The model under review builds one solid part; all positions refer to its coordinate system, in mm. Round coordinates to 2 decimals unless told otherwise and drop trailing zeros. Loops run counter-clockwise (first coordinate to the right, second up) from the corner with the lowest first, then second, coordinate; pieces in that order, holes last. Notation, with made-up numbers: (-14, -24) -> (22, -24) arc R25 ccw to (22, 5) -> close; hole circle Ø10 at (65.5, 55). An arc over 180 degrees is marked (long way). Use CSV: the item, a comma, the result in double quotes. Start each with the question number.
Autodesk Inventor part; units mm, degrees
ref_plane "YZ Plane" through (0, 0, 0) normal (1, 0, 0) x (0, 1, 0)
ref_plane "XZ Plane" through (0, 0, 0) normal (0, 1, 0) x (-1, 0, 0)
ref_plane "XY Plane" through (0, 0, 0) normal (0, 0, 1) x (1, 0, 0)
sketch "Skizze1" plane through (0, 0, 0) normal (1, 0, 0) x (0, 1, 0)
  line L0 (-50, -37.5) -> (50, -37.5)
  line L1 (50, -37.5) -> (50, 37.5)
  line L2 (50, 37.5) -> (-50, 37.5)
  line L3 (-50, 37.5) -> (-50, -37.5)
  line L4 (-50, -37.5) -> (50, 37.5) construction
  line L5 (50, -37.5) -> (-50, 37.5) construction
  point P0 (0, 0)
  dimension "d0" = 100
  dimension "d1" = 75
extrude "Extrusion1" add sketch "Skizze1" along normal blind 0.8
sketch "Skizze2" plane through (0.8, 0, 0) normal (1, 0, 0) x (0, 0, -1)
  line L0 (-37.5, -50) -> (-6.5, -50)
  line L1 (-6.5, -50) -> (-6.5, -44)
  line L2 (-6.5, -44) -> (-37.5, -44)
  line L3 (-37.5, -44) -> (-37.5, -50)
  line L4 (-37.5, 50) -> (-6.5, 50)
  line L5 (-6.5, 50) -> (-6.5, 44)
  line L6 (-6.5, 44) -> (-37.5, 44)
  line L7 (-37.5, 44) -> (-37.5, 50)
  line L8 (31.5, -50) -> (37.5, -50)
  line L9 (37.5, -50) -> (37.5, -44)
  line L10 (37.5, -44) -> (31.5, -44)
  line L11 (31.5, -44) -> (31.5, -50)
  line L12 (37.5, 50) -> (31.5, 50)
  line L13 (31.5, 50) -> (31.5, 44)
  line L14 (31.5, 44) -> (37.5, 44)
  line L15 (37.5, 44) -> (37.5, 50)
  line L16 (-2.5, -37.5) -> (27.5, -37.5)
  line L17 (27.5, -37.5) -> (27.5, 37.5)
  line L18 (27.5, 37.5) -> (-2.5, 37.5)
  line L19 (-2.5, 37.5) -> (-2.5, -37.5)
  line L20 (52.5, 0) -> (-52.5, 0) construction
  line L21 (-37.5, 50) -> (-37.5, -50) construction
  point P0 (0, 0)
  dimension "d4" = 6
  dimension "d5" = 6
  dimension "d6" = 31
  dimension "d9" = 75
  dimension "d10" = 30
  dimension "d11" = 35
extrude "Extrusion2" cut sketch "Skizze2" against normal through all
fillet "Rundung1" radius 6 6 edges at (0.4, -44, 6.5) (0.4, -44, -31.5) (0.4, 44, -31.5) (0.4, 44, 6.5) (0.4, 44, 37.5) (0.4, -44, 37.5)
fillet "Rundung1" radius 0.5 4 edges at (0.4, -37.5, 2.5) (0.4, -37.5, -27.5) (0.4, 37.5, -27.5) (0.4, 37.5, 2.5)
sketch "Skizze3" plane through (0.8, 0, 0) normal (1, 0, 0) x (0, 0, -1)
  line L0 (-37.5, 50) -> (95.7584, 50) construction
  line L1 (95.7584, 50) -> (95.7584, -50) construction
  line L2 (95.7584, -50) -> (-37.5, -50) construction
  line L3 (-37.5, -50) -> (-37.5, 50) construction
  line L4 (-6.5, -50) -> (31.5, -50)
  line L5 (-37.5, 38) -> (-37.5, -38)
  point P0 (0, 0)
  dimension "d26" = 100
decal "Aufkleber1"
sketch "Skizze4" plane through (0.8, 0, 0) normal (1, 0, 0) x (0, 0, -1)
  circle A0 centre (-31, -37.5) radius 1.25
  circle A1 centre (-31, 37.5) radius 1.25
  circle A2 centre (29, -41.5) radius 1.25
  circle A3 centre (29, 41.5) radius 1.25
  line L0 (-37.5, 38) -> (-37.5, -38)
  line L1 (-31.5, -44) -> (-12.5, -44)
  line L2 (52.5, 0) -> (-52.5, 0) construction
  line L3 (-6.5, -50) -> (31.5, -50) construction
  line L4 (37.5, -44) -> (37.5, 44) construction
  point P0 (0, 0)
  dimension "d32" = 6.5
  dimension "d33" = 6.5
  dimension "d34" = 2.5
  dimension "d35" = 8.5
  dimension "d36" = 8.5
extrude "Extrusion3" cut sketch "Skizze4" against normal through all
properties part number "EW_MessingplatteUhrzeit" material "Messing"
1. For line 1 along Y through (x, z) = (0.2, -29); line 2 along Y through (x, z) = (0.5, 31); line 3 along Y through (x, z) = (0.2, -25.5), list the stretches that pass through material, from the lowest coordinate up. Write a range as from..to.
2. Take a section at B-B, the plane z = -14. Give the boundary of the cut face in (x, y).
3. The part is to be moulded in two halves that separate along Z. For faces 1 (the face through (0, -1, 9)), 2 (the face through (0.394, -42.289, 35.696)), 3 (the face through (0.406, 37.021, 29.845)), 4 (the face through (0.41, 42.74, -28.84)), say which applies: pulls with the +Z half, pulls with the -Z half, needs draft (parallel to the pull), parting line crosses it, or undercut.
4. Take a section at C-C, the plane y = -9.5. Give the boundary of the cut face in (x, z), then the cut area to 3 significant figures.
5. Take a section at D-D, the plane x = 0.15. Count the separate pieces of the cut face and the enclosed holes in it, then the cut area to 3 significant figures.
6. Take a section at A-A, the plane z = -29. Give the boundary of the cut face in (x, y), then the cut area to 3 significant figures.
7. Clearance check with a flat-ended pin moving along its axis: P1, Ø2, axis at y = 41.5, z = -29, coming from the +X side. State where the tip first meets the part, or that it passes through.
Results:
1,line 1,"-50..-42.75, -40.25..40.25, 42.75..50"
1,line 2,"-44..-38.75, -36.25..36.25, 38.75..44"
1,line 3,"-50..-37.5, 37.5..50"
2,outline,"(0, -50) -> (0.8, -50) -> (0.8, -37.5) -> (0, -37.5) -> close; (0, 37.5) -> (0.8, 37.5) -> (0.8, 50) -> (0, 50) -> close"
3,face 1,"needs draft"
3,face 2,"pulls with the +Z half"
3,face 3,"undercut"
3,face 4,"undercut"
4,outline,"(0, -37.5) -> (0.8, -37.5) -> (0.8, -27.5) -> (0, -27.5) -> close; (0, 2.5) -> (0.8, 2.5) -> (0.8, 37.5) -> (0, 37.5) -> close"
4,area,"36.0 mm²"
5,separate pieces,"1"
5,enclosed holes,"5"
5,area,"4,800 mm²"
6,outline,"(0, -50) -> (0.8, -50) -> (0.8, -42.75) -> (0, -42.75) -> close; (0, -40.25) -> (0.8, -40.25) -> (0.8, 40.25) -> (0, 40.25) -> close; (0, 42.75) -> (0.8, 42.75) -> (0.8, 50) -> (0, 50) -> close"
6,area,"76.0 mm²"
7,P1,"through"
